The model under review builds one solid part; all positions refer to its coordinate system, in mm. A direction names the side the tool comes from. Coordinates: 2 decimals unless noted, no trailing zeros. Order: outer loops, then holes, each group sorted by start corner. A loop starts at its lowest first (then second) coordinate and runs counter-clockwise, first axis right, second up. Notation, with made-up numbers: M 40,84.5 L 46,84.5 A14 cw 46,110.5 Z; hole C 80,-15.75 d4. An arc over 180 degrees is marked long. Answer as CSV lines item,"result". Start each with the question number.
Q1. Consider section D-D on y = 87.5. Write out the cut boundary in (x, z).
Q2. The part is to be moulded in two halves that separate along X. For faces 1 (the face through (50, 24, -81)), 2 (the face through (49, 100, -51)), 3 (the face through (32.5, 50, -44)), say which applies: +X half, -X half, draft (parallel to the pull), parting line (faces both ways), or undercut.
Q3. Wall thickness on L1, parallel to Y at x = 34.5, z = -47; L2, parallel to Y at x = 50, z = -93.5: over which ranges is each line inside the solid? List them lowest first. Write a range as [from, to].
Q4. Consider section A-A on z = -16.5. Write out the cut boundary in (x, y).
Q5. Consider section C-C on x = 7.5. Write out the cut boundary in (y, z).
Q6. Consider section B-B on y = 50. Write out the cut boundary in (x, z).
Q7. For P1, Ø2.5, axis at x = 63.08, y = 36.92, coming from the -Z side; P2, Ø3, axis at x = 63.08, y = 63.08, coming from the +Z side; P3, Ø8, axis at x = 45, y = 67.5, coming from the -Z side, all flat-tipped, find the tip position at first contact; note any pin that passes through.
Q8. Machinability: for faces 4 (the face through (49, 90, -14)), 5 (the face through (51, 51, -85)), which of the approach directions +Z, -Z, +X, -X, +Y, -Y give a long, thin tool a straight path to every point of the face, cutting with its end or side? Answer none if there is none.
from build123d import *

# Parameters (mm, degrees)
SKETCH_1_W                = 100
SKETCH_1_H                = 100
EXTRUDE_1_DEPTH           = 100
SKETCH_2_R                = 46
CUT_EXTRUDE_1_DEPTH       = 15
FILLET_1_R                = 10
CUT_EXTRUDE_2_DEPTH       = 8
SKETCH_8_W                = 80
SKETCH_8_H                = 80
CUT_EXTRUDE_7_DEPTH       = 28
SKETCH_9_W                = 35
SKETCH_9_H                = 35
CUT_EXTRUDE_8_DEPTH       = 33
SKETCH_10_R               = 2.5
CUT_EXTRUDE_9_DEPTH       = 4
CUT_EXTRUDE_10_DEPTH      = 163.975458275
CUT_EXTRUDE_10_DEPTH_BACK = 20
SKETCH_11_R               = 1


with BuildPart() as part:
    # 草图1 → 凸台-拉伸1 (new body)
    with BuildSketch(Plane(origin=(0, 0, 0), x_dir=(1, 0, 0), z_dir=(0, 1, 0))):
        with Locations((50, 50)):
            Rectangle(SKETCH_1_W, SKETCH_1_H)
    extrude(amount=EXTRUDE_1_DEPTH)

    # 草图2 → 切除-拉伸1 (cut)
    with BuildSketch(Plane(origin=(0, 0, -100), x_dir=(-1, 0, 0), z_dir=(0, 0, -1))):
        with Locations((-50, 50)):
            Circle(SKETCH_2_R)
    extrude(amount=-CUT_EXTRUDE_1_DEPTH, mode=Mode.SUBTRACT)

    # 圆角1
    fillet_1_edges = [part.edges().sort_by_distance(p)[0] for p in [
        (100, 100, -50),
        (0, 100, -50),
        (100, 0, -50),
        (0, 0, -50),
    ]]
    fillet(fillet_1_edges, radius=FILLET_1_R)

    # 草图3 → 切除-拉伸2 (cut)
    with BuildSketch(Plane(origin=(0, 0, -85), x_dir=(-1, 0, 0), z_dir=(0, 0, -1))):
        with BuildLine():
            Line((-61.860285343, 26.862722036), (-69.615087298, 11.734501829))
            ThreePointArc((-69.615087298, 11.734501829), (-50, 7), (-30.384912702, 11.734501829))
            Line((-30.384912702, 11.734501829), (-38.139714657, 26.862722036))
            ThreePointArc((-38.139714657, 26.862722036), (-50, 24), (-61.860285343, 26.862722036))
        make_face()
    extrude(amount=-CUT_EXTRUDE_2_DEPTH, mode=Mode.SUBTRACT)

    # 草图6 → section 1 of loft_1
    with BuildSketch(Plane(origin=(0, 0, -65), x_dir=(-1, 0, 0), z_dir=(0, 0, -1)), mode=Mode.PRIVATE) as loft_1_s1:
        with BuildLine():
            Line((-69.615087298, 11.734501829), (-65.965768731, 18.853664279))
            ThreePointArc((-65.965768731, 18.853664279), (-50, 15), (-34.034231269, 18.853664279))
            Line((-34.034231269, 18.853664279), (-30.384912702, 11.734501829))
            ThreePointArc((-30.384912702, 11.734501829), (-50, 7), (-69.615087298, 11.734501829))
        make_face()
    # loft from a face of the part (loft_1)
    loft([part.faces().sort_by_distance((50, 16.103496225, -77))[0], loft_1_s1.sketch], mode=Mode.SUBTRACT)

    # 草图6<3> for 切除-放样3 → 切除-放样3 section 0
    with BuildSketch(Plane(origin=(0, 0, -65), x_dir=(-1, 0, 0), z_dir=(0, 0, -1))):
        with BuildLine():
            Line((-69.615087298, 11.734501829), (-65.965768731, 18.853664279))
            # circular arc as an exact rational Bezier (weights 1, cos(half-angle), 1)
            Bezier((-65.965768731, 18.853664279), (-50, 10.669530728), (-34.034231269, 18.853664279), weights=[1, 0.889895306, 1])
            Line((-34.034231269, 18.853664279), (-30.384912702, 11.734501829))
            Bezier((-30.384912702, 11.734501829), (-50, 1.67970918), (-69.615087298, 11.734501829), weights=[1, 0.889895306, 1])
        make_face()
    # 草图7 → 切除-放样3 section 1
    with BuildSketch(Plane.XZ):
        with BuildLine():
            Line((65.965768731, -60.646196457), (34.034231269, -60.646196457))
            Line((34.034231269, -60.646196457), (38.139714657, -45.646196457))
            Line((38.139714657, -45.646196457), (61.860285343, -45.646196457))
            Line((61.860285343, -45.646196457), (65.965768731, -60.646196457))
        make_face()
    loft(mode=Mode.SUBTRACT)

    # 草图8 → 切除-拉伸7 (cut)
    with BuildSketch(Plane.XY):
        with Locations((50, 50)):
            Rectangle(SKETCH_8_W, SKETCH_8_H)
    extrude(amount=-CUT_EXTRUDE_7_DEPTH, mode=Mode.SUBTRACT)

    # 草图9 → 切除-拉伸8 (cut)
    with BuildSketch(Plane.XY.offset(-28)):
        with Locations((50, 50)):
            Rectangle(SKETCH_9_W, SKETCH_9_H)
    extrude(amount=-CUT_EXTRUDE_8_DEPTH, mode=Mode.SUBTRACT)

    # 草图10 → 切除-拉伸9 (cut)
    with BuildSketch(Plane(origin=(0, 0, -85), x_dir=(-1, 0, 0), z_dir=(0, 0, -1))):
        with Locations((-36.918524548, 36.918524548)):
            Circle(SKETCH_10_R)
        with Locations(Location((-36.918524548, 63.081475452, 0), (0, 0, 180))):
            Circle(SKETCH_10_R)
        with Locations(Location((-63.081475452, 36.918524548, 0), (0, 0, 180))):
            Circle(SKETCH_10_R)
        with Locations((-63.081475452, 63.081475452)):
            Circle(SKETCH_10_R)
    extrude(amount=-CUT_EXTRUDE_9_DEPTH, mode=Mode.SUBTRACT)

    # 草图11 → 切除-拉伸10 (cut, two sides: drawn at the far end of the back side and taken through both)
    with BuildSketch(Plane(origin=(0, 0, -81), x_dir=(-1, 0, 0), z_dir=(0, 0, -1)).offset(-CUT_EXTRUDE_10_DEPTH_BACK)):
        with Locations((-63.081475452, 63.081475452)):
            Circle(SKETCH_11_R)
        with Locations(Location((-36.918524548, 63.081475452, 0), (0, 0, 180))):
            Circle(SKETCH_11_R)
        with Locations(Location((-63.081475452, 36.918524548, 0), (0, 0, 180))):
            Circle(SKETCH_11_R)
        with Locations((-36.918524548, 36.918524548)):
            Circle(SKETCH_11_R)
    extrude(amount=CUT_EXTRUDE_10_DEPTH + CUT_EXTRUDE_10_DEPTH_BACK, mode=Mode.SUBTRACT)


solid = part.part
Evaluation:
1,outline,"M 0,-100 L 23.36,-100 L 23.36,-85 L 76.64,-85 L 76.64,-100 L 100,-100 L 100,0 L 90,0 L 90,-28 L 10,-28 L 10,0 L 0,0 Z"
2,face 1,"undercut"
2,face 2,"draft"
2,face 3,"undercut"
3,L1,"y = [0, 32.5], [67.5, 100]"
3,L2,"y = [0, 4], [96, 100]"
4,outline,"M 0,10 A10 ccw 10,0 L 90,0 A10 ccw 100,10 L 100,90 A10 ccw 90,100 L 10,100 A10 ccw 0,90 Z; hole M 10,10 L 90,10 L 90,90 L 10,90 Z"
5,outline,"M 0.32,-100 L 32.4,-100 L 32.4,-85 L 67.6,-85 L 67.6,-100 L 99.68,-100 L 99.68,0 L 0.32,0 Z"
6,outline,"M 0,-100 L 4,-100 L 4,-85 L 96,-85 L 96,-100 L 100,-100 L 100,0 L 90,0 L 90,-28 L 67.5,-28 L 67.5,-61 L 32.5,-61 L 32.5,-28 L 10,-28 L 10,0 L 0,0 Z"
7,P1,"stops at z = -81"
7,P2,"stops at z = -61"
7,P3,"stops at z = -85"
8,face 4,"+Z"
8,face 5,"-Z"
